Source: three-view drawing plus pictorial views. Frame: mm from the lowest corner of the part. A direction names the side the tool comes from. Coordinates: 2 decimals unless noted, no trailing zeros. Order: outer loops, then holes, each group sorted by start corner. A loop starts at its lowest first (then second) coordinate and runs counter-clockwise, first axis right, second up. Notation, with made-up numbers: (64, -9) -> (110, -9) arc R24 cw to (110, 8) -> close; hole circle Ø3 at (55, 82.25). An arc over 180 degrees is marked (long way). Use one line per item in the form item = value. Start each with the question number.
1) Section query C-C on x = 38.5. Output: boundary loops of the cut face in (y, z).
2) Access query for the marked faces 1 and 2. Directions: +Z, -Z, +X, -X, +Y, -Y. A direction counts if a zero-diameter tool reaches every point of the face in a straight line with its end or side. Return the directions, or none.
3) Section query A-A on y = 3.5. Output: boundary loops of the cut face in (x, z).
4) Ray query, line 1 along Z through (x, y) = (36.5, 23); line 2 along X through (y, z) = (13.5, 35.5). Return the intervals inside material, ascending.
5) Pin query (flat end, axial travel): pin 1 (1 mm diameter, centred on y = 12, z = 23.5, fed in from +X); pin 2 (14.5 mm diameter, centred on x = 47, y = 11.5, fed in from +Z). Return the tip coordinate at first contact, or that it passes through.
6) Section query B-B on z = 30. Output: boundary loops of the cut face in (x, y).
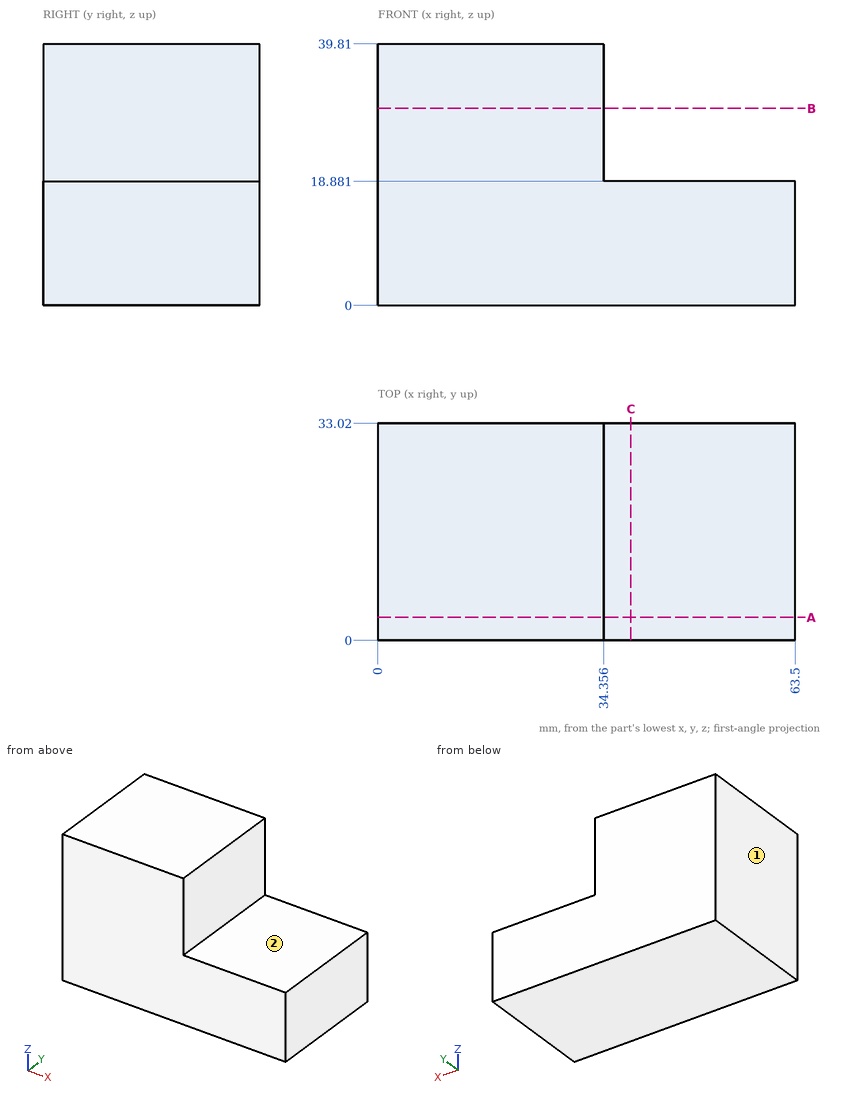
Answers below:
q1.outline = (0, 0) -> (33.02, 0) -> (33.02, 18.88) -> (0, 18.88) -> close
q2.face_1 = +Z, -Z, -X, +Y, -Y
q2.face_2 = +Z, +X, +Y, -Y
q3.outline = (0, 0) -> (63.5, 0) -> (63.5, 18.88) -> (34.36, 18.88) -> (34.36, 39.81) -> (0, 39.81) -> close
q4.line_1 = 0 to 18.88
q4.line_2 = 0 to 34.36
q5.pin_1 = 34.36
q5.pin_2 = 18.88
q6.outline = (0, 0) -> (34.36, 0) -> (34.36, 33.02) -> (0, 33.02) -> close
